Here's how the part is built. I have some questions about the finished solid (model axes, mm). Coordinates: 2 decimals unless noted, no trailing zeros. Order: outer loops, then holes, each group sorted by start corner. A loop starts at its lowest first (then second) coordinate and runs counter-clockwise, first axis right, second up. Notation, with made-up numbers: (21, -14.75) -> (54, -14.75) arc R20 ccw to (54, -1.75) -> close; hole circle Ø4 at (1, -30). An arc over 180 degrees is marked (long way). One line per item, written item: value. Start each with the question number.
```python
from build123d import *

# Parameters (mm, degrees)
SZKIC1_R                    = 100
SZKIC1_R_2                  = 75
SZKIC1_R_3                  = 3.4
DODANIE_WYCI_GNI_CIE1_DEPTH = 10
SFAZOWANIE1_SIZE            = 2


with BuildPart() as part:
    # Szkic1 → Dodanie-wyciągnięcie1 (new, symmetric)
    with BuildSketch(Plane.XY):
        Circle(SZKIC1_R)
        Circle(SZKIC1_R_2, mode=Mode.SUBTRACT)
        with Locations((0, 87.5)):
            Circle(SZKIC1_R_3, mode=Mode.SUBTRACT)
        with Locations((87.5, 0)):
            Circle(SZKIC1_R_3, mode=Mode.SUBTRACT)
        with Locations((0, -87.5)):
            Circle(SZKIC1_R_3, mode=Mode.SUBTRACT)
        with Locations((-87.5, 0)):
            Circle(SZKIC1_R_3, mode=Mode.SUBTRACT)
    extrude(amount=DODANIE_WYCI_GNI_CIE1_DEPTH, both=True)

    # Sfazowanie1
    sfazowanie1_edges = [part.edges().sort_by_distance(p)[0] for p in [
        (-100, 0, -10),
    ]]
    chamfer(sfazowanie1_edges, length=SFAZOWANIE1_SIZE)


solid = part.part
```
Q1. If we mould it in two halves opening along X, with no side actions, what happens to faces 1 (the face through (95.38, 30.04, 1.13)), 2 (the face through (22, -74, 10)), 3 (the face through (-9.764, 74.362, -0.14))? For each: +X half, -X half, draft (parallel to the pull), parting line (faces both ways), or undercut.
Q2. I need wall thicknesses on line 1 (Y direction, x = 0, z = -2.25); line 2 (X direction, y = 69.5, z = -1.75); line 3 (Y direction, x = -22, z = -8.5). Which ranges of each line are inside material? Lowest first, please.
Q3. Imagine slicing it at A-A (x = 0). Write out the boundary of the cut face in (y, z), plus the area to 3 significant figures.
Q4. Imagine slicing it at C-C (z = 6.75). Write out the boundary of the cut face in (x, y).
Q5. For P1, Ø10, axis at x = 22, z = 7, coming from the +Y side; P2, Ø2, axis at x = 62.5, z = -1, coming from the +Y side; P3, Ø1.5, axis at y = -30.5, z = 7, coming from the -X side; P4, Ø6, axis at x = 87.5, y = 0, coming from the +Z side, each with a flat end and sliding along its axis, tell me the tip position at first contact or that it passes through.
Completed:
1. face 1: parting line
1. face 2: draft
1. face 3: undercut
2. line 1: y = -100 to -90.9, -84.1 to -75, 75 to 84.1, 90.9 to 100
2. line 2: x = -71.9 to -28.19, 28.19 to 71.9
2. line 3: y = -97.04 to -71.7, 71.7 to 97.04
3. outline: (-100, -8) -> (-98, -10) -> (-90.9, -10) -> (-90.9, 10) -> (-100, 10) -> close; (-84.1, -10) -> (-75, -10) -> (-75, 10) -> (-84.1, 10) -> close; (75, -10) -> (84.1, -10) -> (84.1, 10) -> (75, 10) -> close; (90.9, -10) -> (98, -10) -> (100, -8) -> (100, 10) -> (90.9, 10) -> close
3. area: 724 mm2
4. outline: circle Ø200 at (0, 0); hole circle Ø6.8 at (-87.5, 0); hole circle Ø150 at (0, 0); hole circle Ø6.8 at (0, -87.5); hole circle Ø6.8 at (0, 87.5); hole circle Ø6.8 at (87.5, 0)
5. P1: stops at y = 98.54
5. P2: stops at y = 78.85
5. P3: stops at x = -95.47
5. P4: passes through
